Design review of the part built by this model. Coordinates are the model's own, in mm. A direction names the side the tool comes from. Coordinates: 2 decimals unless noted, no trailing zeros. Loops run counter-clockwise (first coordinate to the right, second up) from the corner with the lowest first, then second, coordinate; pieces in that order, holes last. Notation, with made-up numbers: M 74.25,-37.75 L 83.25,-37.75 A23 ccw 83.25,-23.75 Z; hole C 5,43 d9. An arc over 180 degrees is marked long. Put each result on its own line as item: value. Start each with the question number.
(1) The part is to be moulded in two halves that separate along Z. For faces 1 (the cylindrical face through (20.636, -1.565, 0.132)), 2 (the cylindrical face through (-16.506, -1.565, 0.168)), 3 (the cylindrical face through (0.356, -1.851, -21.192)), 4 (the flat face through (0, -3.175, -3)), say which applies: +Z half, -Z half, draft (parallel to the pull), parting line (faces both ways), or undercut.
(2) For probe 1 along Y at (x, z) = (5.5, 5.5) (3 decimals); probe 2 along Z at (x, y) = (-12.7, -1); probe 3 along Z at (x, y) = (-12.7, -2.25), list the stretches that pass through material, from the lowest coordinate up. Write a range as [from, to].
(3) Clearance check with flat-ended pins moving along their axes: pin 1 (10 mm diameter, centred on x = -12.7, z = 0, fed in from +Y); pin 2 (1.5 mm diameter, centred on x = 19.5, y = 15.5, fed in from +Z); pin 3 (8 mm diameter, centred on x = 13, y = 11, fed in from +Z). State where each tip first meets the part, or that it passes through.
(4) Take a section at A-A, the plane z = 0. Give the boundary of the cut face in (x, y) (1 decimal), then the cut area to 3 significant figures.
(5) Take a section at C-C, the plane z = 6. Give the boundary of the cut face in (x, y) (3 decimals).
(6) Take a section at D-D, the plane x = -6.5. Give the boundary of the cut face in (y, z) (3 decimals).
(7) For faces 5 (the flat face through (25.4, -1, -9)), 6 (the cylindrical face through (4.764, -1.565, -0.132)), 7 (the flat face through (0, 0, -1)), list the 3-axis set-ups (+Z, -Z, +X, -X, +Y, -Y) from which the entire face can be reached by the end or side of a thin tool; tool diameter is ignored.
(8) Take a section at B-B, the plane x = -12.7. Give the boundary of the cut face in (y, z) (3 decimals).
```python
from build123d import *

# Parameters (mm, degrees)
F0_W     = 50.8
F0_H     = 31.75
F0_R     = 1.5875
F0_R_2   = 3.81
F1_DEPTH = 3.175
F3_DEPTH = 50.8
F4_R     = 2.54
F5_R     = 2.54


with BuildPart() as f1:
    # F0 (on Front) → F1 (new body)
    with BuildSketch(Plane.XZ):
        with Locations((0, -3.175)):
            Rectangle(F0_W, F0_H)
        with Locations((-20.828, 0)):
            Circle(F0_R, mode=Mode.SUBTRACT)
        with Locations((-12.7, 0)):
            Circle(F0_R_2, mode=Mode.SUBTRACT)
        with BuildLine():
            ThreePointArc((9.7426447204, -7.366), (4.7625, 0), (9.7426447204, 7.366))
            Line((9.7426447204, 7.366), (15.6573552796, 7.366))
            ThreePointArc((15.6573552796, 7.366), (20.6375, 0), (15.6573552796, -7.366))
            Line((15.6573552796, -7.366), (9.7426447204, -7.366))
        make_face(mode=Mode.SUBTRACT)
    extrude(amount=F1_DEPTH)

    # F2 (on face) → F3 (join, through all)
    with BuildSketch(Plane(origin=(-25.4, 0, 0), x_dir=(0, -1, 0), z_dir=(-1, 0, 0))):
        Polygon((2.3532495318, -22.1168144985), (3.175, -19.05), (-23.7399423715, -11.8381629272), (-24.5616928397, -14.9049774257), align=None)
    extrude(amount=-F3_DEPTH)

    # F4
    f4_edges = [f1.edges().sort_by_distance(p)[0] for p in [
        (0, 0, -18.199261),
    ]]
    fillet(f4_edges, radius=F4_R)

    # F5
    f5_edges = [f1.edges().sort_by_distance(p)[0] for p in [
        (0, -2.35325, -22.116814),
        (0, -3.175, -19.05),
    ]]
    fillet(f5_edges, radius=F5_R)


solid = f1.part
```
Computed values:
1. face 1: undercut
1. face 2: undercut
1. face 3: -Z half
1. face 4: draft
2. probe 1: y = [-3.175, 0]
2. probe 2: z = [-21.51, -3.81], [3.81, 12.7]
2. probe 3: z = [-20.9, -3.81], [3.81, 12.7]
3. pin 1: stops at y = 0
3. pin 2: stops at z = -13.85
3. pin 3: stops at z = -14.18
4. outline: M -25.4,-3.2 L -22.4,-3.2 L -22.4,0 L -25.4,0 Z; M -19.2,-3.2 L -16.5,-3.2 L -16.5,0 L -19.2,0 Z; M -8.9,-3.2 L 4.8,-3.2 L 4.8,0 L -8.9,0 Z; M 20.6,-3.2 L 25.4,-3.2 L 25.4,0 L 20.6,0 Z
4. area: 76.6 mm^2
5. outline: M -25.4,-3.175 L 7.503,-3.175 L 7.503,0 L -25.4,0 Z; M 17.897,-3.175 L 25.4,-3.175 L 25.4,0 L 17.897,0 Z
6. outline: M -3.175,-18.716 A2.54 ccw -3.088,-19.373 L -3.011,-19.663 A2.54 ccw 0.1,-21.459 L 24.562,-14.905 L 23.74,-11.838 L 3.197,-17.343 A2.54 cw 0,-14.889 L 0,12.7 L -3.175,12.7 Z
7. face 5: +Z, -Z, +X, +Y, -Y
7. face 6: +Y, -Y
7. face 7: +Z, +X, -X
8. outline: M -3.175,-18.716 A2.54 ccw -3.088,-19.373 L -3.011,-19.663 A2.54 ccw 0.1,-21.459 L 24.562,-14.905 L 23.74,-11.838 L 3.197,-17.343 A2.54 cw 0,-14.889 L 0,-3.81 L -3.175,-3.81 Z; M -3.175,3.81 L 0,3.81 L 0,12.7 L -3.175,12.7 Z
